from build123d import *

# Parameters (mm, degrees)
SKETCH1_W           = 5
SKETCH1_H           = 20
SKETCH1_W_2         = 20
SKETCH1_H_2         = 5
BOSS_EXTRUDE2_DEPTH = 50
BOSS_EXTRUDE3_DEPTH = 2
BOSS_EXTRUDE4_DEPTH = 1
SKETCH5_W           = 10.627555573
SKETCH5_H           = 30
CUT_EXTRUDE1_DEPTH  = 410
SKETCH6_R           = 9.876593792
BOSS_EXTRUDE5_DEPTH = 4


with BuildPart() as part:
    # Sketch1 → Boss-Extrude2 (new body)
    with BuildSketch(Plane(origin=(0, 0, 0), x_dir=(0, 0, -1), z_dir=(1, 0, 0))):
        with Locations((11.964285714, 8.526785714)):
            Rectangle(SKETCH1_W, SKETCH1_H)
        with Locations((4.464285714, 21.026785714)):
            Rectangle(SKETCH1_W_2, SKETCH1_H_2)
        with Locations((4.464285714, -3.973214286)):
            Rectangle(SKETCH1_W_2, SKETCH1_H_2)
    extrude(amount=BOSS_EXTRUDE2_DEPTH)

    # Sketch2 → Boss-Extrude3 (add)
    with BuildSketch(Plane.XZ.offset(-18.526785714)):
        with BuildLine():
            Line((4.515759803, -9.464285714), (4.515759803, 5.535714286))
            add(Edge.make_bspline(
                [(4.515759803, 5.535714286), (5.848786982, -3.806136343), (13.48902105, -9.464285714)],
                knots=[0, 0, 0, 1, 1, 1], degree=2))
            Line((13.48902105, -9.464285714), (4.515759803, -9.464285714))
        make_face()
    extrude(amount=BOSS_EXTRUDE3_DEPTH)

    # Sketch4 → Boss-Extrude4 (add)
    with BuildSketch(Plane.XZ.offset(-18.526785714)):
        with BuildLine():
            Line((17.865518754, -10.317847861), (17.865518754, 5.535714286))
            add(Edge.make_bspline(
                [(17.865518754, 5.535714286), (18.795797839, -4.399262704), (26.838780001, -10.317847861)],
                knots=[0, 0, 0, 1, 1, 1], degree=2))
            Line((26.838780001, -10.317847861), (17.865518754, -10.317847861))
        make_face()
    extrude(amount=BOSS_EXTRUDE4_DEPTH)

    # Sketch5 → Cut-Extrude1 (cut)
    with BuildSketch(Plane(origin=(50, 0, 0), x_dir=(0, 0, -1), z_dir=(1, 0, 0))):
        with Locations((-0.221936499, 8.526785714)):
            Rectangle(SKETCH5_W, SKETCH5_H)
    extrude(amount=-CUT_EXTRUDE1_DEPTH, mode=Mode.SUBTRACT)

    # Sketch6 → Boss-Extrude5 (add)
    with BuildSketch(Plane.XY.offset(-9.464285714)):
        with Locations(Location((38.269602277, 8.445873505, 0), (0, 0, 90))):
            Circle(SKETCH6_R)
    extrude(amount=BOSS_EXTRUDE5_DEPTH)


solid = part.part
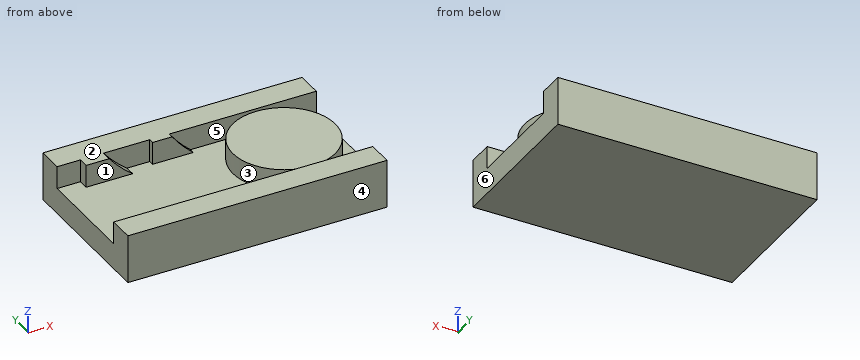
For this review, take the finished solid that the model builds, in its own axes (mm). Face numbers are marked on the shaded views. A direction names the side the tool comes from. Round coordinates to 2 decimals unless told otherwise and drop trailing zeros. Loops run counter-clockwise (first coordinate to the right, second up) from the corner with the lowest first, then second, coordinate; pieces in that order, holes last. Notation, with made-up numbers: (-33.75, -9.5) - (11.25, -9.5) arc R9 cw to (11.25, -0.5) - close; hole circle Ø11 at (36.5, 19). An arc over 180 degrees is marked (long way). Use one line per item in the form item = value.
Item 1: Tool access review of the marked faces 1, 2 and 3: name each direction out of +Z, -Z, +X, -X, +Y, -Y from which nothing blocks a thin tool from reaching the whole face with its end or side.
Answers:
face_1 = +Z, -X
face_2 = +Z, +X, -X, +Y, -Y
face_3 = +Z
Item 2: Consider section D-D on x = 34.5. Write out the cut boundary in (y, z).
Answers:
outline = (-6.47, -14.46) - (23.53, -14.46) - (23.53, -5.09) - (18.53, -5.09) - (18.53, -9.46) - (17.57, -9.46) - (17.57, -5.46) - (-0.68, -5.46) - (-0.68, -9.46) - (-1.47, -9.46) - (-1.47, -5.09) - (-6.47, -5.09) - close
Item 3: Consider section C-C on z = -6.5. State how many separate pieces and enclosed holes the cut face has, then the cut area to 3 significant figures.
Answers:
separate_pieces = 3
enclosed_holes = 0
area = 823 mm^2
Item 4: Mouldability with a two-part tool opening along Y and no side actions: class the marked faces 4, 5 and 6 as +Y half, -Y half, draft (parallel to the pull), parting line (faces both ways), or undercut.
Answers:
face_4 = -Y half
face_5 = undercut
face_6 = draft
Item 5: Consider section A-A on x = 20. Write out the cut boundary in (y, z).
Answers:
outline = (-6.47, -14.46) - (23.53, -14.46) - (23.53, -5.09) - (17.53, -5.09) - (17.53, -9.46) - (-1.47, -9.46) - (-1.47, -5.09) - (-6.47, -5.09) - close
Item 6: Consider section B-B on y = 8. Write out the cut boundary in (x, z).
Answers:
outline = (0, -14.46) - (50, -14.46) - (50, -9.46) - (48.14, -9.46) - (48.14, -5.46) - (28.4, -5.46) - (28.4, -9.46) - (0, -9.46) - close
Item 7: For line 1 (Y direction, x = 27, z = -5.75); line 2 (Y direction, x = 42.5, z = -6); line 3 (Z direction, x = 44, y = 0), list the stretches that pass through material, from the lowest coordinate up.
Answers:
line_1 = -6.47 to -1.47, 18.53 to 23.53
line_2 = -6.47 to -1.47, -0.48 to 17.37, 18.53 to 23.53
line_3 = -14.46 to -9.46
Item 8: Clearance check with flat-ended pins moving along their axes: P1, Ø0.5, axis at y = 18, z = -8, coming from the -X side; P2, Ø2, axis at y = 18, z = -7, coming from the -X side; P3, Ø6, axis at x = 41.5, y = 3.5, coming from the +Z side. State where each tip first meets the part, or that it passes through.
Answers:
P1 = 4.52
P2 = 0
P3 = -5.46
